The model under review builds one solid part; all positions refer to its coordinate system, in mm. A direction names the side the tool comes from. Round coordinates to 2 decimals unless told otherwise and drop trailing zeros. Write each loop counter-clockwise with the first axis right and the second up, starting at its lowest first coordinate (ties: lowest second). Pieces come first, ordered by that corner, then holes. Notation, with made-up numbers: (61.5, -18.75) - (104.5, -18.75) arc R24 cw to (104.5, 12.25) - close; hole circle Ø6 at (34, 40). An arc over 180 degrees is marked (long way). Write each question's results on one line, items separated by ' | '.
```python
from build123d import *

# Parameters (mm, degrees)
SKETCH1_R           = 14
BOSS_EXTRUDE1_DEPTH = 28
SKETCH2_R           = 1.5
CUT_EXTRUDE1_DEPTH  = 4
SKETCH5_R           = 1.5
BOSS_EXTRUDE2_DEPTH = 20


with BuildPart() as part:
    # Sketch1 → Boss-Extrude1 (new body)
    with BuildSketch(Plane(origin=(0, 0, 0), x_dir=(1, 0, 0), z_dir=(0, 1, 0))):
        with Locations(Location((0, 0, 0), (0, 0, 270))):
            Circle(SKETCH1_R)
    extrude(amount=BOSS_EXTRUDE1_DEPTH)

    # Sketch2 → Cut-Extrude1 (cut)
    with BuildSketch(Plane.XZ):
        with Locations(Location((0, 8, 0), (0, 0, 270))):
            Circle(SKETCH2_R)
        with Locations(Location((9.5, 0, 0), (0, 0, 270))):
            Circle(SKETCH2_R)
        with Locations(Location((0, -8, 0), (0, 0, 270))):
            Circle(SKETCH2_R)
        with Locations(Location((-9.5, 0, 0), (0, 0, 270))):
            Circle(SKETCH2_R)
    extrude(amount=-CUT_EXTRUDE1_DEPTH, mode=Mode.SUBTRACT)

    # Sketch4 → Cut-Revolve1 (revolve, cut)
    with BuildSketch(Plane.XY, mode=Mode.PRIVATE) as cut_revolve1_sk:
        with BuildLine():
            Line((-14, 23), (-14, 28))
            Line((-14, 28), (-4, 28))
            Line((-4, 28), (-4, 27))
            ThreePointArc((-4, 27), (-9.385164807, 25.962912018), (-14, 23))
        make_face()
    revolve(cut_revolve1_sk.sketch.rotate(Axis((0, 28, 0), (0, -1, 0)), 270), axis=Axis((0, 28, 0), (0, -1, 0)), mode=Mode.SUBTRACT)

    # Sketch5 → Boss-Extrude2 (add)
    with BuildSketch(Plane(origin=(0, 28, 0), x_dir=(1, 0, 0), z_dir=(0, 1, 0))):
        with Locations(Location((0, 0, 0), (0, 0, 270))):
            Circle(SKETCH5_R)
    extrude(amount=BOSS_EXTRUDE2_DEPTH)


solid = part.part
```
Q1. The part is to be moulded in two halves that separate along Z. For faces 4 (the cylindrical face through (-11, 2, 0)), 5 (the flat face through (0, 48, 0)), 6 (the cylindrical face through (-13.67, 11.34, -3.03)), say which applies: released by +Z, released by -Z, zero draft, split by the parting line, or undercut.
Evaluation:
face 4: undercut | face 5: zero draft | face 6: split by the parting line
Q2. Tool access review of faces 1 (the cylindrical face through (3.905, 27.493, -0.867)), 2 (the cylindrical face through (0.07, 1.97, -6.5)), 3 (the flat face through (0, 0, 0)): name each direction out of +Z, -Z, +X, -X, +Y, -Y from which nothing blocks a thin tool from reaching the whole face with its end or side.
Evaluation:
face 1: +Y | face 2: -Y | face 3: +Z, -Z, +X, -X, -Y
Q3. Insertion check: P1, Ø2, axis at x = -10, y = 14.5, coming from the +Z side; P2, Ø5, axis at y = 15, z = 4.5, coming from the +X side; P3, Ø0.9, axis at x = -0.5, z = -8.5, coming from the -Y side. Each pin has a flat end and moves straight along its axis. Give the tip position at first contact, or say it passes through.
Evaluation:
P1: stops at z = 10.72 | P2: stops at x = 13.86 | P3: stops at y = 4
Q4. We need section A-A (y = 42). State the section outline as (x, z) points, plus the area to 3 significant figures.
Evaluation:
outline: circle Ø3 at (0, 0) | area: 7.07 mm^2
Q5. We need section B-B (y = 12). State the section outline as (x, z) points.
Evaluation:
outline: circle Ø28 at (0, 0)
Q6. For probe 1 along X at (y, z) = (1.1, 0); probe 2 along X at (y, z) = (8.5, -2.75); probe 3 along X at (y, z) = (4, 5.5), list the stretches that pass through material, from the lowest coordinate up.
Evaluation:
probe 1: x = -14 to -11, -8 to 8, 11 to 14 | probe 2: x = -13.73 to 13.73 | probe 3: x = -12.87 to 12.87
